Geometry check sheet. Reference: the model listing, model coordinates, mm. Face numbers are marked on the shaded views. A direction names the side the tool comes from. Give positions to 0.01 mm unless a question says otherwise; leave off trailing zeros. Order: outer loops, then holes, each group sorted by start corner. A loop starts at its lowest first (then second) coordinate and runs counter-clockwise, first axis right, second up. Notation, with made-up numbers: (36, 40.5) - (48, 40.5) arc R19 cw to (48, 62.5) - close; hole circle Ø2 at (18.25, 33). An arc over 180 degrees is marked (long way). Put each result on its own line as item: value. Start each with the question number.
```python
from build123d import *

# Parameters (mm, degrees)
SKETCH1_W               = 16
SKETCH1_H               = 39.5
BOSS_EXTRUDE1_DEPTH     = 15
SKETCH2_W               = 10
SKETCH2_H               = 33.5
CUT_EXTRUDE1_DEPTH      = 3
CUT_EXTRUDE2_DEPTH      = 45.274710615
CUT_EXTRUDE2_DEPTH_BACK = 45.274710615
SKETCH3_R               = 1.6
CUT_EXTRUDE3_DEPTH      = 3
CUT_EXTRUDE3_DEPTH_BACK = 46.180194776
SKETCH4_R               = 1.6
SKETCH5_R               = 2.5
CUT_EXTRUDE4_DEPTH      = 20
SKETCH7_R               = 4.25
CUT_EXTRUDE5_DEPTH      = 4


with BuildPart() as part:
    # Sketch1 → Boss-Extrude1 (new body)
    with BuildSketch(Plane(origin=(0, 0, 0), x_dir=(1, 0, 0), z_dir=(0, 1, 0))):
        with Locations((8, 19.75)):
            Rectangle(SKETCH1_W, SKETCH1_H)
    extrude(amount=BOSS_EXTRUDE1_DEPTH)

    # Sketch2 → Cut-Extrude1 (cut)
    with BuildSketch(Plane(origin=(0, 15, 0), x_dir=(1, 0, 0), z_dir=(0, 1, 0))):
        with Locations((8, 19.75)):
            Rectangle(SKETCH2_W, SKETCH2_H)
    extrude(amount=-CUT_EXTRUDE1_DEPTH, mode=Mode.SUBTRACT)

    # Sketch3 → Cut-Extrude2 (cut, two sides: drawn at the far end of the back side and taken through both)
    with BuildSketch(Plane(origin=(0, 12, 0), x_dir=(1, 0, 0), z_dir=(0, 1, 0)).offset(-CUT_EXTRUDE2_DEPTH_BACK)):
        with Locations(Location((2.7, 2.5, 0), (0, 0, 270))):
            Circle(SKETCH3_R)
    extrude(amount=CUT_EXTRUDE2_DEPTH + CUT_EXTRUDE2_DEPTH_BACK, mode=Mode.SUBTRACT)

    # Sketch4 → Cut-Extrude3 (cut, two sides: drawn at the far end of the back side and taken through both)
    with BuildSketch(Plane(origin=(0, 15, 0), x_dir=(1, 0, 0), z_dir=(0, 1, 0)).offset(-CUT_EXTRUDE3_DEPTH_BACK)):
        with Locations(Location((13.3, 2.5, 0), (0, 0, 100.806922875))):
            Circle(SKETCH4_R)
        with Locations(Location((2.7, 17, 0), (0, 0, 79.193077125))):
            Circle(SKETCH4_R)
        with Locations(Location((2.5, 36, 0), (0, 0, 18.209956864))):
            Circle(SKETCH4_R)
    extrude(amount=CUT_EXTRUDE3_DEPTH + CUT_EXTRUDE3_DEPTH_BACK, mode=Mode.SUBTRACT)

    # Sketch5 → Cut-Extrude4 (cut)
    with BuildSketch(Plane(origin=(0, 12, 0), x_dir=(1, 0, 0), z_dir=(0, 1, 0))):
        with Locations(Location((8, 26, 0), (0, 0, 270))):
            Circle(SKETCH5_R)
    extrude(amount=-CUT_EXTRUDE4_DEPTH, mode=Mode.SUBTRACT)

    # Sketch7 → Cut-Extrude5 (cut)
    with BuildSketch(Plane(origin=(0, 12, 0), x_dir=(1, 0, 0), z_dir=(0, 1, 0))):
        with Locations(Location((8, 26, 0), (0, 0, 270))):
            Circle(SKETCH7_R)
    extrude(amount=-CUT_EXTRUDE5_DEPTH, mode=Mode.SUBTRACT)


solid = part.part
```
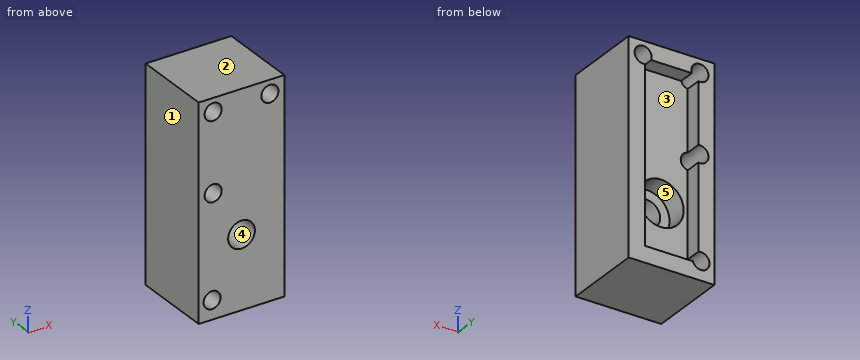
Item 1: Cross-section at A-A (z = -36). Enter the section's corners in (x, y), and give its area (3 significant figures).
Item 2: Cross-section at D-D (x = 7.5). Enter the section's corners in (y, z).
Item 3: Set-up check for the marked faces 4 and 5: record each of +Z, -Z, +X, -X, +Y, -Y from which the full face is reachable in a straight line by a thin tool's end or side.
Item 4: Cross-section at C-C (y = 4.75). Enter the section's corners in (x, z).
Item 5: Thickness scan on line 1 along X through (y, z) = (3, -26); line 2 along X through (y, z) = (7, -36); line 3 along Z through (x, y) = (2.5, 3.5). Record the ranges inside material, lowest first.
Item 6: Release check for a two-part mould opening along X. For the marked faces 1, 2 and 3 record: +X half, -X half, draft (parallel to the pull), parting line (faces both ways), or undercut.
Item 7: Gauge pin test, flat end, axial feed: pin 1 Ø1.9 at (x, z) = (2.5, -36) entering from -Y. Record the tip position at first contact, or that the pin passes through.
Item 8: Cross-section at B-B (z = -2.5). Enter the section's corners in (x, y).
Recorded:
1. outline: (0, 0) - (0.9, 0) - (0.9, 15) - (0, 15) - close; (4.1, 0) - (16, 0) - (16, 15) - (13, 15) - (13, 12) - (4.1, 12) - close
1. area: 165 mm^2
2. outline: (0, -39.5) - (15, -39.5) - (15, -36.5) - (12, -36.5) - (12, -30.22) - (8, -30.22) - (8, -28.45) - (0, -28.45) - close; (0, -23.55) - (8, -23.55) - (8, -21.78) - (12, -21.78) - (12, -3) - (15, -3) - (15, 0) - (0, 0) - close
3. face 4: +Y, -Y
3. face 5: +Y
4. outline: (0, -39.5) - (16, -39.5) - (16, 0) - (0, 0) - close; hole circle Ø3.2 at (2.5, -36); hole circle Ø3.2 at (2.7, -17); hole circle Ø3.2 at (2.7, -2.5); hole circle Ø5 at (8, -26); hole circle Ø3.2 at (13.3, -2.5)
5. line 1: x = 0 to 5.5, 10.5 to 16
5. line 2: x = 0 to 0.9, 4.1 to 16
5. line 3: z = -39.5 to -37.6, -34.4 to -18.59, -15.41 to -4.09, -0.91 to 0
6. face 1: -X half
6. face 2: draft
6. face 3: undercut
7. pin 1: passes through
8. outline: (0, 0) - (1.1, 0) - (1.1, 15) - (0, 15) - close; (4.3, 0) - (11.7, 0) - (11.7, 15) - (4.3, 15) - close; (14.9, 0) - (16, 0) - (16, 15) - (14.9, 15) - close
